Can you work these out from the model? Positions are in its coordinate system, mm. Round coordinates to 2 decimals unless told otherwise and drop trailing zeros. Use CSV: the item, a comma, the result in double quotes.
```python
from build123d import *

# Parameters (mm, degrees)
F0_W     = 302
F0_H     = 38
F0_W_2   = 8
F0_H_2   = 16
F1_DEPTH = 2.5
F2_D     = 2.5
F3_D     = 4.5
F4_DEPTH = 2.501


with BuildPart() as f1:
    # F0 (on Top) → F1 (new body)
    with BuildSketch(Plane.XY):
        Rectangle(F0_W, F0_H)
        with Locations((-136, 0)):
            Rectangle(F0_W_2, F0_H_2, mode=Mode.SUBTRACT)
        with Locations((-120, 0)):
            Rectangle(F0_W_2, F0_H_2, mode=Mode.SUBTRACT)
        with Locations((-104, 0)):
            Rectangle(F0_W_2, F0_H_2, mode=Mode.SUBTRACT)
        with Locations((-88, 0)):
            Rectangle(F0_W_2, F0_H_2, mode=Mode.SUBTRACT)
        with Locations((-72, 0)):
            Rectangle(F0_W_2, F0_H_2, mode=Mode.SUBTRACT)
        with Locations((-56, 0)):
            Rectangle(F0_W_2, F0_H_2, mode=Mode.SUBTRACT)
        with Locations((-40, 0)):
            Rectangle(F0_W_2, F0_H_2, mode=Mode.SUBTRACT)
        with Locations((-24, 0)):
            Rectangle(F0_W_2, F0_H_2, mode=Mode.SUBTRACT)
        with Locations((-8, 0)):
            Rectangle(F0_W_2, F0_H_2, mode=Mode.SUBTRACT)
        with Locations((8, 0)):
            Rectangle(F0_W_2, F0_H_2, mode=Mode.SUBTRACT)
        with Locations((24, 0)):
            Rectangle(F0_W_2, F0_H_2, mode=Mode.SUBTRACT)
        with Locations((40, 0)):
            Rectangle(F0_W_2, F0_H_2, mode=Mode.SUBTRACT)
        with Locations((56, 0)):
            Rectangle(F0_W_2, F0_H_2, mode=Mode.SUBTRACT)
        with Locations((72, 0)):
            Rectangle(F0_W_2, F0_H_2, mode=Mode.SUBTRACT)
        with Locations((88, 0)):
            Rectangle(F0_W_2, F0_H_2, mode=Mode.SUBTRACT)
        with Locations((104, 0)):
            Rectangle(F0_W_2, F0_H_2, mode=Mode.SUBTRACT)
        with Locations((120, 0)):
            Rectangle(F0_W_2, F0_H_2, mode=Mode.SUBTRACT)
        with Locations((136, 0)):
            Rectangle(F0_W_2, F0_H_2, mode=Mode.SUBTRACT)
    extrude(amount=-F1_DEPTH)

    # F2 (through all)
    with Locations(Plane.XY):
        with Locations((-128, 0), (-96, 0), (-64, 0), (-32, 0), (0, 0), (32, 0), (64, 0), (96, 0), (128, 0)):
            Hole(F2_D / 2)

    # F3 (through all)
    with Locations(Plane.XY):
        with Locations((-146, 14), (-146, -14), (146, 14), (146, -14)):
            Hole(F3_D / 2)

    # F0 (on Top) → F4 (cut, through all)
    with BuildSketch(Plane.XY):
        with Locations((-136, 0)):
            Rectangle(F0_W_2, F0_H_2)
    extrude(amount=-F4_DEPTH, mode=Mode.SUBTRACT)


solid = f1.part
```
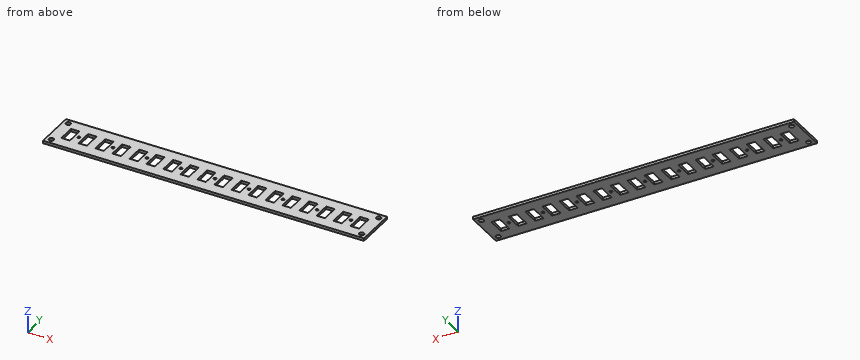
Q1. Please list where these lines run through material, in increasing order: probe 1 along Y at (x, z) = (146, -1.1); probe 2 along Y at (x, z) = (-128, -0.6); probe 3 along Y at (x, z) = (91.5, -2.3).
Resolved:
probe 1,"y = -19 to -16.25, -11.75 to 11.75, 16.25 to 19"
probe 2,"y = -19 to -1.25, 1.25 to 19"
probe 3,"y = -19 to -8, 8 to 19"
Q2. Suppose I cut it at A-A (z = -0.7). Count the separate pieces of the cut face and the enclosed holes in it, and give its area (3 significant figures).
Resolved:
separate pieces,"1"
enclosed holes,"31"
area,"9,060 mm^2"
Q3. Will this pin go through, and if not, where does the flat tip stop? P1, Ø7, axis at x = 146, y = -14, coming from the +Z side.
Resolved:
P1,"stops at z = 0"
